Design review of the part built by this model. Coordinates are the model's own, in mm. A direction names the side the tool comes from. Coordinates: 2 decimals unless noted, no trailing zeros. Write each loop counter-clockwise with the first axis right and the second up, starting at its lowest first coordinate (ties: lowest second). Pieces come first, ordered by that corner, then holes.
Q1. Clearance check with flat-ended pins moving along their axes: pin 1 Ø19 at (x, y) = (138, 3.5) entering from -Z; pin 2 Ø6.5 at (x, z) = (132.5, -567.5) entering from +Y; pin 3 Ø11.5 at (x, y) = (123, -7) entering from +Z. State where each tip first meets the part, or that it passes through.
Q2. Machinability: for faces 1 (the face through (139, 0, 774.7)), 2 (the face through (139, 0, -571.5)), 3 (the face through (139, 0, 520.7)), which of the approach directions +Z, -Z, +X, -X, +Y, -Y give a long, thin tool a straight path to every point of the face, cutting with its end or side? Answer none if there is none.
Q3. Add section B-B, the plane z = 435.5. Give the boundary of the cut face in (x, y), plus the area to 3 significant figures.
Q4. Add section A-A, the plane y = -75. Give the boundary of the cut face in (x, z).
Q5. To check wall thickness, follow probe 1 along Y at (x, z) = (158, 768); probe 2 along X at (y, z) = (25, -250). State the ranges of each line that lie inside material, in increasing order.
from build123d import *

# Parameters (mm, degrees)
F0_W     = 203.2
F0_H     = 1727.2
F1_DEPTH = 101.6
F2_W     = 38.1
F2_H     = 12.7
F3_DEPTH = 76.2
F4_R     = 19.04999
F5_R     = 9.525
F6_DEPTH = 1638.301


# Not quite as in the source:
# - a fillet or chamfer is up to 0.001 mm smaller than in the source, because OpenCascade refuses the exact size


with BuildPart() as f1:
    # F0 (on Front) → F1 (new body, symmetric)
    with BuildSketch(Plane.XZ):
        Rectangle(F0_W, F0_H)
    extrude(amount=F1_DEPTH, both=True)

    # F2 (on face) → F3 (join)
    with BuildSketch(Plane.YZ.offset(101.6)):
        with Locations((0, -565.15)):
            Rectangle(F2_W, F2_H)
        with Locations((0, -323.85)):
            Rectangle(F2_W, F2_H)
        with Locations((0, 527.05)):
            Rectangle(F2_W, F2_H)
        with Locations((0, 768.35)):
            Rectangle(F2_W, F2_H)
    extrude(amount=F3_DEPTH)

    # F4 (radius 19.05 in the source; OpenCascade refuses exactly that, so slightly less here)
    f4_edges = [f1.edges().sort_by_distance(p)[0] for p in [
        (177.8, 19.05, -565.15),
        (177.8, -19.05, -565.15),
        (177.8, 19.05, -323.85),
        (177.8, -19.05, -323.85),
        (177.8, 19.05, 527.05),
        (177.8, -19.05, 527.05),
        (177.8, 19.05, 768.35),
        (177.8, -19.05, 768.35),
    ]]
    fillet(f4_edges, radius=F4_R)

    # F5 (on face) → F6 (cut, through all)
    with BuildSketch(Plane.XY.offset(774.7)):
        with Locations((158.75, 0)):
            Circle(F5_R)
    extrude(amount=-F6_DEPTH, mode=Mode.SUBTRACT)


solid = f1.part
Here are the results:
1. pin 1: stops at z = -571.5
1. pin 2: stops at y = 19.05
1. pin 3: stops at z = 774.7
2. face 1: +Z, +X, +Y, -Y
2. face 2: -Z, +X, +Y, -Y
2. face 3: +X, +Y, -Y
3. outline: (-101.6, -101.6) - (101.6, -101.6) - (101.6, 101.6) - (-101.6, 101.6) - close
3. area: 41,300 mm2
4. outline: (-101.6, -863.6) - (101.6, -863.6) - (101.6, 863.6) - (-101.6, 863.6) - close
5. probe 1: y = -19.05 to -9.5, 9.5 to 19.05
5. probe 2: x = -101.6 to 101.6
